Verification items for the finished model (mm, model axes). Face numbers are marked on the shaded views. Round coordinates to 2 decimals unless told otherwise and drop trailing zeros. Loops run counter-clockwise (first coordinate to the right, second up) from the corner with the lowest first, then second, coordinate; pieces in that order, holes last. Notation, with made-up numbers: (82, 52.5) - (94, 52.5) arc R35 cw to (94, 89.5) - close; hole circle Ø9 at (24, 80.25). An arc over 180 degrees is marked (long way). Use CSV: the item, a comma, the result in double quotes.
```python
from build123d import *

# Parameters (mm, degrees)
SKETCH_1_W          = 12.5
SKETCH_1_H          = 28.5
EXTRUDE_1_DEPTH     = 7.5
SKETCH_2_W          = 3
SKETCH_2_H          = 28.488787575
EXTRUDE_2_DEPTH     = 5
SKETCH_3_R          = 11.5
CUT_EXTRUDE_1_DEPTH = 1
SKETCH_4_R          = 12.5
CUT_EXTRUDE_2_DEPTH = 4
SKETCH_5_R          = 10.75
CUT_EXTRUDE_3_DEPTH = 0.5
SKETCH_6_R          = 10
CUT_EXTRUDE_4_DEPTH = 1
SKETCH_7_W          = 18
SKETCH_7_H          = 18
CUT_EXTRUDE_5_DEPTH = 1
EXTRUDE_5_DEPTH     = 1


with BuildPart() as part:
    # 草图1 → 凸台-拉伸1 (new body)
    with BuildSketch(Plane.XY):
        Rectangle(SKETCH_1_W, SKETCH_1_H)
    extrude(amount=EXTRUDE_1_DEPTH)

    # 草图2 → 凸台-拉伸2 (add)
    with BuildSketch(Plane.XY.offset(7.5)):
        with Locations((-4.75, 0.005606212)):
            Rectangle(SKETCH_2_W, SKETCH_2_H)
    extrude(amount=EXTRUDE_2_DEPTH)

    # 草图3 → 切除-拉伸1 (cut)
    with BuildSketch(Plane(origin=(0, 0, 0), x_dir=(-1, 0, 0), z_dir=(0, 0, -1))):
        with Locations((-7.75, 0)):
            Circle(SKETCH_3_R)
    extrude(amount=-CUT_EXTRUDE_1_DEPTH, mode=Mode.SUBTRACT)

    # 草图4 → 切除-拉伸2 (cut)
    with BuildSketch(Plane(origin=(0, 0, 1), x_dir=(-1, 0, 0), z_dir=(0, 0, -1))):
        with Locations((-7.75, 0)):
            Circle(SKETCH_4_R)
    extrude(amount=-CUT_EXTRUDE_2_DEPTH, mode=Mode.SUBTRACT)

    # 草图5 → 切除-拉伸3 (cut)
    with BuildSketch(Plane(origin=(0, 0, 5), x_dir=(-1, 0, 0), z_dir=(0, 0, -1))):
        with Locations((-7.75, 0)):
            Circle(SKETCH_5_R)
    extrude(amount=-CUT_EXTRUDE_3_DEPTH, mode=Mode.SUBTRACT)

    # 草图6 → 切除-拉伸4 (cut)
    with BuildSketch(Plane(origin=(0, 0, 5.5), x_dir=(-1, 0, 0), z_dir=(0, 0, -1))):
        with Locations((-7.75, 0)):
            Circle(SKETCH_6_R)
    extrude(amount=-CUT_EXTRUDE_4_DEPTH, mode=Mode.SUBTRACT)

    # 草图7 → 切除-拉伸5 (cut)
    with BuildSketch(Plane(origin=(0, 0, 6.5), x_dir=(-1, 0, 0), z_dir=(0, 0, -1))):
        with Locations((-7.75, 0)):
            Rectangle(SKETCH_7_W, SKETCH_7_H)
    extrude(amount=-CUT_EXTRUDE_5_DEPTH, mode=Mode.SUBTRACT)

    # 草图9 → 凸台-拉伸5 (add)
    with BuildSketch(Plane.XY.offset(6.5)):
        with BuildLine():
            Line((3.391101056, 9), (-1.25, 9))
            Line((-1.25, 9), (-1.25, 4.358898944))
            ThreePointArc((-1.25, 4.358898944), (0.678932188, 7.071067812), (3.391101056, 9))
        make_face()
        with BuildLine():
            Line((-1.25, -4.358898944), (-1.25, -9))
            Line((-1.25, -9), (3.391101056, -9))
            ThreePointArc((3.391101056, -9), (0.678932188, -7.071067812), (-1.25, -4.358898944))
        make_face()
    extrude(amount=EXTRUDE_5_DEPTH)


solid = part.part
```
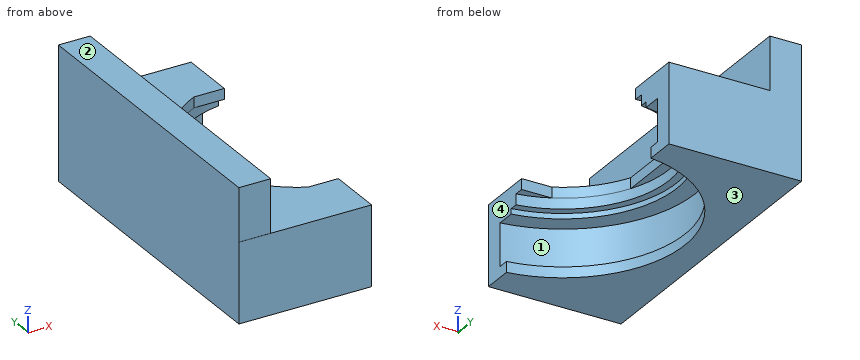
1) Cross-section at B-B, the plane y = 7.75. Record the cut outline in (x, z).
Returned:
outline,"(-6.25, 0) - (-0.75, 0) - (-0.75, 1) - (-2.06, 1) - (-2.06, 5) - (0.3, 5) - (0.3, 5.5) - (1.43, 5.5) - (1.43, 7.5) - (-3.25, 7.5) - (-3.25, 12.5) - (-6.25, 12.5) - close"
2) Cross-section at A-A, the plane x = -0.25. Record the cut outline in (y, z), then the cut area to 3 significant figures.
Returned:
outline,"(-14.25, 0) - (-8.26, 0) - (-8.26, 1) - (-9.6, 1) - (-9.6, 5) - (-7.18, 5) - (-7.18, 5.5) - (-6, 5.5) - (-6, 7.5) - (-14.25, 7.5) - close; (6, 5.5) - (7.18, 5.5) - (7.18, 5) - (9.6, 5) - (9.6, 1) - (8.26, 1) - (8.26, 0) - (14.25, 0) - (14.25, 7.5) - (6, 7.5) - close"
area,"89.2 mm²"
3) Mould release check, pull along Z, two halves, no side actions. Record for the marked faces 1, 2, 3 and 4: +Z half, -Z half, draft (parallel to the pull), parting line (faces both ways), or undercut.
Returned:
face 1,"undercut"
face 2,"+Z half"
face 3,"-Z half"
face 4,"draft"
4) Thickness scan on probe 1 along Z at (x, y) = (-4.25, 2.75); probe 2 along X at (y, z) = (0, 4); probe 3 along Z at (x, y) = (-1.5, 0.25). Record the ranges inside material, lowest first. Write a range as [from, to].
Returned:
probe 1,"z = [0, 1], [5, 12.5]"
probe 2,"x = [-6.25, -4.75]"
probe 3,"z = [6.5, 7.5]"
5) Cross-section at C-C, the plane z = 6. Record the cut outline in (x, y).
Returned:
outline,"(-6.25, -14.25) - (6.25, -14.25) - (6.25, -9.89) arc R10 cw to (6.25, 9.89) - (6.25, 14.25) - (-6.25, 14.25) - close"
6) Cross-section at D-D, the plane x = 3. Record the cut outline in (y, z).
Returned:
outline,"(-14.25, 0) - (-10.47, 0) - (-10.47, 1) - (-11.56, 1) - (-11.56, 5) - (-9.64, 5) - (-9.64, 5.5) - (-8.8, 5.5) - (-8.8, 7.5) - (-14.25, 7.5) - close; (8.8, 5.5) - (9.64, 5.5) - (9.64, 5) - (11.56, 5) - (11.56, 1) - (10.47, 1) - (10.47, 0) - (14.25, 0) - (14.25, 7.5) - (8.8, 7.5) - close"
7) Gauge pin test, flat ends, axial feed: pin 1 Ø1.5 at (x, y) = (-1, -8.5) entering from +Z; pin 2 Ø1.1 at (y, z) = (-0.5, 7) entering from +X; pin 3 Ø3.5 at (x, z) = (-5.5, 9.5) entering from -Y. Record the tip position at first contact, or that the pin passes through.
Returned:
pin 1,"stops at z = 7.5"
pin 2,"stops at x = -1.25"
pin 3,"stops at y = -14.24"
